from build123d import *

# Parameters (mm, degrees)
CROQUIS1_W              = 4
CROQUIS1_H              = 14
CROQUIS1_R              = 1.5
SALIENTE_EXTRUIR1_DEPTH = 3
CROQUIS2_W              = 6
CROQUIS2_H              = 3.5
SALIENTE_EXTRUIR2_DEPTH = 10
SALIENTE_EXTRUIR3_START = -3
CROQUIS3_R              = 5
CROQUIS3_R_2            = 1.5
SALIENTE_EXTRUIR3_DEPTH = 3
REDONDEO1_R             = 3


# Read off the part's stored shape, not the designer's step: TaladroAvanzado1
with BuildPart() as part:
    # Croquis1 → Saliente-Extruir1 (new body)
    with BuildSketch(Plane(origin=(0, 0, 0), x_dir=(1, 0, 0), z_dir=(0, 1, 0))):
        with Locations((2, 7)):
            Rectangle(CROQUIS1_W, CROQUIS1_H)
        with Locations(Location((2, 2, 0), (0, 0, 270))):
            Circle(CROQUIS1_R, mode=Mode.SUBTRACT)
    extrude(amount=SALIENTE_EXTRUIR1_DEPTH)

    # Croquis2 → Saliente-Extruir2 (add)
    with BuildSketch(Plane(origin=(0, 3, 0), x_dir=(1, 0, 0), z_dir=(0, 1, 0))):
        with Locations((3, 15.75)):
            Rectangle(CROQUIS2_W, CROQUIS2_H)
    extrude(amount=-SALIENTE_EXTRUIR2_DEPTH)

    # Croquis3 → Saliente-Extruir3 (add)
    with BuildSketch(Plane(origin=(0, 3, 0), x_dir=(1, 0, 0), z_dir=(0, 1, 0)).offset(SALIENTE_EXTRUIR3_START)):
        with Locations((2, 2)):
            Circle(CROQUIS3_R)
        with Locations(Location((2, 2, 0), (0, 0, 270))):
            Circle(CROQUIS3_R_2, mode=Mode.SUBTRACT)
    extrude(amount=SALIENTE_EXTRUIR3_DEPTH)

    # TaladroAvanzado1 outline → TaladroAvanzado1 (revolve, cut)
    with BuildSketch(Plane(origin=(2, 0, -2), x_dir=(1, 0, 0), z_dir=(0, 0, 1))):
        Polygon((1.5, 1.34), (1.7, 1.34), (3.36, 3), (1.5, 3), align=None)
    revolve(axis=Axis((2, 0, -2), (0, 1, 0)), mode=Mode.SUBTRACT)

    # Redondeo1
    # the kernel refuses this fillet: 3 mm, written as the material it adds along each edge
    with BuildSketch(Plane(origin=(4, 0, -14), x_dir=(1, 0, 0), z_dir=(0, 1, 0))) as redondeo1_piece_1:
        with BuildLine():
            CenterArc((3, -2.828427125), REDONDEO1_R, 109.471220634, 70.528779366)
            Line((0, -2.828427125), (-0.06, -2.828427125))
            Line((-0.06, -2.828427125), (-0.06, 0))
            Line((-0.06, 0), (0, 0.06))
            ThreePointArc((0, 0.06), (1, 0.06), (1.98, 0.056568542))
            Line((1.98, 0.056568542), (2, 0))
        make_face()
    extrude(amount=3)
    with BuildSketch(Plane(origin=(4, 3, -6.582575695), x_dir=(0, 0, -1), z_dir=(0, -1, 0))) as redondeo1_piece_2:
        with BuildLine():
            CenterArc((1.662422303, 3), REDONDEO1_R, 218.682187453, 51.317812547)
            Line((-0.679451946, 1.125), (-0.726289431, 1.0875))
            ThreePointArc((-0.726289431, 1.0875), (-0.353961086, 0.5539026), (-0.054990908, -0.024))
            Line((-0.054990908, -0.024), (0, -0.06))
            Line((0, -0.06), (1.662422303, -0.06))
            Line((1.662422303, -0.06), (1.662422303, 0))
        make_face()
    extrude(amount=3)
    with BuildSketch(Plane(origin=(0, 3, -6.582575695), x_dir=(0, 0, -1), z_dir=(0, -1, 0))) as redondeo1_piece_3:
        with BuildLine():
            CenterArc((1.662422303, -3), REDONDEO1_R, 90, 51.317812547)
            Line((-0.679451946, -1.125), (-0.726289431, -1.0875))
            ThreePointArc((-0.726289431, -1.0875), (-0.353961086, -0.5539026), (-0.054990908, 0.024))
            Line((-0.054990908, 0.024), (0, 0.06))
            Line((0, 0.06), (1.662422303, 0.06))
            Line((1.662422303, 0.06), (1.662422303, 0))
        make_face()
    extrude(amount=3)


solid = part.part
Geometry check sheet. Reference: the model listing, model coordinates, mm. A direction names the side the tool comes from. Round coordinates to 2 decimals unless told otherwise and drop trailing zeros. Order: outer loops, then holes, each group sorted by start corner. A loop starts at its lowest first (then second) coordinate and runs counter-clockwise, first axis right, second up. Notation, with made-up numbers: M -32.75,84.5 L -23.75,84.5 A23 ccw -23.75,103.5 Z; hole C 19.25,28 d10. An arc over 180 degrees is marked long. Answer in a Markdown table with one row per item.
(1) Sectioned sample at A-A, the plane x = 2. Record the cut outline in (y, z), and give its area (3 significant figures).
Responses:
| item | result |
|---|---|
| outline | M -7,-17.5 L 3,-17.5 L 3,-5.36 L 1.34,-3.7 L 1.34,-3.5 L 0,-3.5 L 0,-14 L -7,-14 Z; M 0,-0.5 L 1.34,-0.5 L 1.34,-0.3 L 3,1.36 L 3,3 L 0,3 Z |
| area | 73.6 mm² |
(2) Scan lines: probe 1 along X at (y, z) = (1.05, -2); probe 2 along Z at (x, y) = (2, 0.8); probe 3 along Y at (x, z) = (-0.75, -4.5). Record each from-to range of solid material in increasing order. Write a range as from..to.
Responses:
| item | result |
|---|---|
| probe 1 | x = -3..0.5, 3.5..7 |
| probe 2 | z = -17.5..-3.5, -0.5..3 |
| probe 3 | y = 0..3 |
(3) Draft check along Z on faces 1 (the face through (3, -3, -14)), 2 (the face through (1.425, 0.661, -0.614)), 3 (the face through (0, -1, -15)). Enter one of: released by +Z, released by -Z, zero draft, split by the parting line, or undercut.
Responses:
| item | result |
|---|---|
| face 1 | released by +Z |
| face 2 | undercut |
| face 3 | zero draft |
(4) Go/stop test with flat-tipped pins: P1, Ø4, axis at x = 2.5, z = -10.5, coming from the -Y side; P2, Ø3.5, axis at x = 2.5, z = -2, coming from the +Y side; P3, Ø3, axis at y = 1, z = -6.5, coming from the +X side. Record where each tip stops, or that it passes through.
Responses:
| item | result |
|---|---|
| P1 | stops at y = 0 |
| P2 | stops at y = 1.89 |
| P3 | stops at x = 6 |
(5) Sectioned sample at D-D, the plane y = -2.25. Record the cut outline in (x, z).
Responses:
| item | result |
|---|---|
| outline | M 0,-17.5 L 6,-17.5 L 6,-14 L 0,-14 Z |
(6) Sectioned sample at B-B, the plane z = -2. Record the cut outline in (x, y).
Responses:
| item | result |
|---|---|
| outline | M -3,0 L 0.5,0 L 0.5,1.34 L 0.3,1.34 L -1.36,3 L -3,3 Z; M 3.5,0 L 7,0 L 7,3 L 5.36,3 L 3.7,1.34 L 3.5,1.34 Z |
(7) Sectioned sample at C-C, the plane z = -15.5. Record the cut outline in (x, y).
Responses:
| item | result |
|---|---|
| outline | M 0,-7 L 6,-7 L 6,3 L 0,3 Z |
(8) Tool access check on faces 4 (the face through (4.304, 1.521, -6.929)), 5 (the face through (3, -2, -17.5)), 6 (the face through (6, -2, -16)), 7 (the face through (2, 0, -4)). Record the directions out of +Z, -Z, +X, -X, +Y, -Y that give a thin tool (end or side, any length) a straight path to the whole face; none if there is none.
Responses:
| item | result |
|---|---|
| face 4 | +X, +Y, -Y |
| face 5 | -Z, +X, -X, +Y, -Y |
| face 6 | -Z, +X, +Y, -Y |
| face 7 | +Z, +X, -X, -Y |
